from build123d import *

# Parameters (mm, degrees)
F0_W = 2
F0_H = 2


# Not quite as in the source:
# - a feature names something its author has since deleted; it is built from what else it names


with BuildPart() as f1:
    # F0 (on Front) → F1 (revolve)
    with BuildSketch(Plane.XZ):
        with Locations((5, 14)):
            Rectangle(F0_W, F0_H)
        Polygon((4, 13), (4, 15), (3, 20), (2, 20), (3, 0), (4, 0), align=None)
        Polygon((3, 20), (4, 15), (6, 15), align=None)
    revolve(axis=Axis((0, 0, 10.5782048777), (0, 0, 1)))


solid = f1.part
For this review, take the finished solid that the model builds, in its own axes (mm). A direction names the side the tool comes from. Coordinates: 2 decimals unless noted, no trailing zeros. Loops run counter-clockwise (first coordinate to the right, second up) from the corner with the lowest first, then second, coordinate; pieces in that order, holes last. Notation, with made-up numbers: (8, -23.5) -> (28, -23.5) arc R20 ccw to (28, -5.5) -> close; hole circle Ø1 at (24.5, -4). An arc over 180 degrees is marked (long way). Write each question's results on one line, items separated by ' | '.
Q1. Add section A-A, the plane y = 0. State the section outline as (x, z) points, then the cut area to 3 significant figures.
Taken from the geometry:
outline: (-6, 13) -> (-4, 13) -> (-4, 0) -> (-3, 0) -> (-2, 20) -> (-3, 20) -> (-6, 15) -> close; (2, 20) -> (3, 0) -> (4, 0) -> (4, 13) -> (6, 13) -> (6, 15) -> (3, 20) -> close | area: 73.0 mm²
Q2. For pin 1 Ø3 at (x, z) = (-2, 8.5) entering from +Y; pin 2 Ø2 at (x, z) = (2.5, 6) entering from -Y; pin 3 Ø1 at (y, z) = (-2, 15.5) entering from +X, all flat-tipped, find the tip position at first contact; note any pin that passes through.
Taken from the geometry:
pin 1: y = 3.97 | pin 2: y = -3.71 | pin 3: x = 5.7
Q3. To check wall thickness, follow line 1 along X through (y, z) = (0.5, 1.5); line 2 along Y through (x, z) = (1.5, 16); line 3 along Y through (x, z) = (-0.75, 13.75). State the ranges of each line that lie inside material, in increasing order. Write a range as [from, to].
Taken from the geometry:
line 1: [-3.97, -2.88], [2.88, 3.97] | line 2: [-5.19, -1.61], [1.61, 5.19] | line 3: [-5.95, -2.19], [2.19, 5.95]
Q4. Mouldability with a two-part tool opening along Y and no side actions: class faces 3 (the conical face through (2.391, 0.753, 9.86)), 4 (the flat face through (-1, 3, 0)), 5 (the cylindrical face through (-0.867, -3.905, 6.591)) as +Y half, -Y half, draft (parallel to the pull), parting line (faces both ways), or undercut.
Taken from the geometry:
face 3: undercut | face 4: draft | face 5: parting line
Q5. Add section D-D, the plane z = 11.5. State the section outline as (x, y) points (3 decimals).
Taken from the geometry:
outline: circle Ø8 at (0, 0); hole circle Ø4.85 at (0, 0)
Q6. Machinability: for faces 1 (the flat face through (1.42, -3.92, 13)), 2 (the flat face through (1, -2, 20)), which of the approach directions +Z, -Z, +X, -X, +Y, -Y give a long, thin tool a straight path to every point of the face, cutting with its end or side? Answer none if there is none.
Taken from the geometry:
face 1: -Z | face 2: +Z, +X, -X, +Y, -Y
Q7. Add section C-C, the plane z = 3. State the section outline as (x, y) points, then the cut area to 3 significant figures.
Taken from the geometry:
outline: circle Ø8 at (0, 0); hole circle Ø5.7 at (0, 0) | area: 24.7 mm²
